Geometry: see drawing. Coordinates: mm, zero at the bounding-box minimum. Coordinates: 2 decimals unless noted, no trailing zeros. Order: outer loops, then holes, each group sorted by start corner. A loop starts at its lowest first (then second) coordinate and runs counter-clockwise, first axis right, second up.
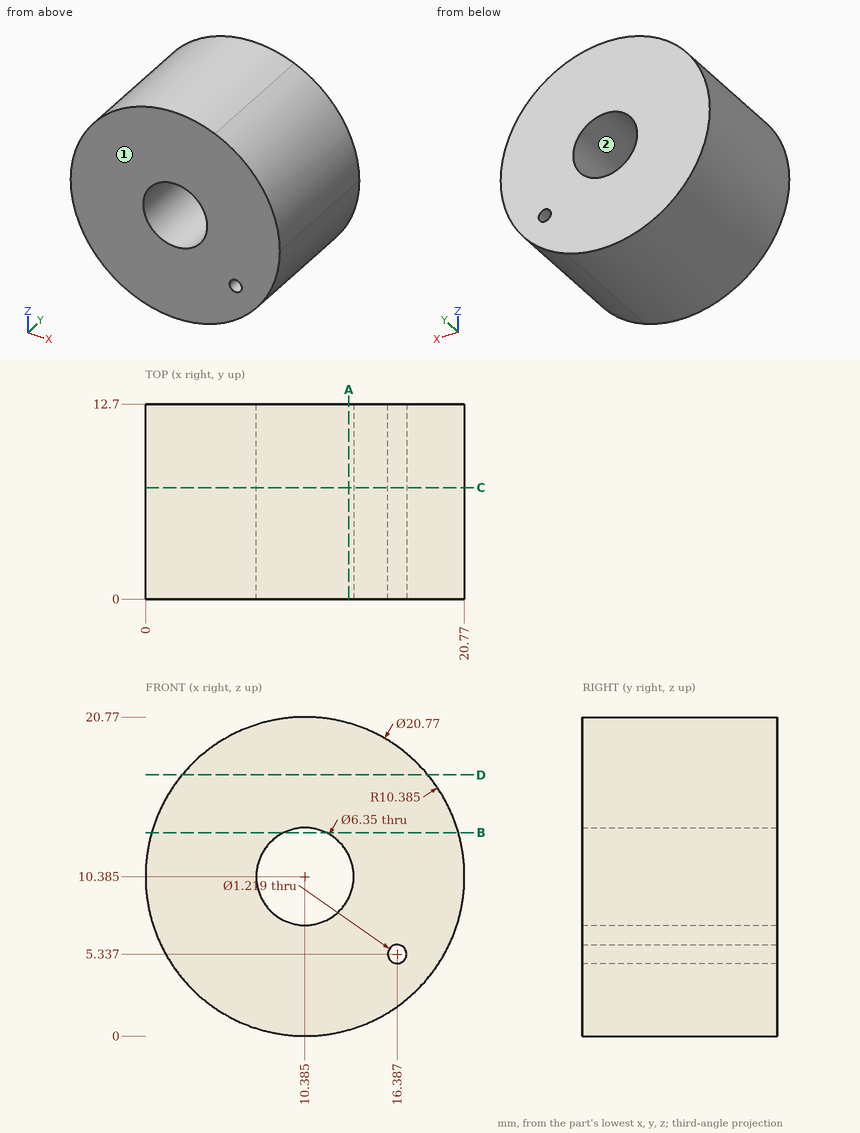
Item 1: Ray query, probe 1 along Z at (x, y) = (10.5, 10.5); probe 2 along X at (y, z) = (2.5, 11.25) (1 decimal). Return the intervals inside material, ascending.
Response values:
probe 1: z = 0 to 7.21, 13.56 to 20.77
probe 2: x = 0 to 7.3, 13.4 to 20.7
Item 2: Draft query along X for the marked faces 1 and 2. Return one class per face: pulls with the +X half, pulls with the -X half, needs draft (parallel to the pull), parting line crosses it, or undercut.
Response values:
face 1: needs draft
face 2: undercut
Item 3: Cut plane B-B on z = 13.25. Return loops of the section in (x, y).
Response values:
outline: (0.4, 0) - (9.02, 0) - (9.02, 12.7) - (0.4, 12.7) - close; (11.75, 0) - (20.37, 0) - (20.37, 12.7) - (11.75, 12.7) - close
Item 4: Cut plane A-A on x = 13.25. Return loops of the section in (y, z), then the cut area to 3 significant figures.
Response values:
outline: (0, 0.4) - (12.7, 0.4) - (12.7, 9.02) - (0, 9.02) - close; (0, 11.75) - (12.7, 11.75) - (12.7, 20.37) - (0, 20.37) - close
area: 219 mm2
Item 5: Cut plane C-C on y = 7.25. Count the separate pieces of the cut face and the enclosed holes in it, then the cut area to 3 significant figures.
Response values:
separate pieces: 1
enclosed holes: 2
area: 306 mm2
Item 6: Pin query (flat end, axial travel): pin 1 Ø4 at (y, z) = (3.5, 15) entering from -X (1 decimal); pin 2 Ø3 at (x, y) = (17.5, 6.5) entering from -Z; pin 3 Ø4 at (y, z) = (2, 17.5) entering from -X. Return the tip coordinate at first contact, or that it passes through.
Response values:
pin 1: stops at x = 0.3
pin 2: stops at z = 1.65
pin 3: stops at x = 1.35
Item 7: Cut plane D-D on z = 17. Return loops of the section in (x, y), then the cut area to 3 significant figures.
Response values:
outline: (2.38, 0) - (18.39, 0) - (18.39, 12.7) - (2.38, 12.7) - close
area: 203 mm2
